```python
from build123d import *

# Parameters (mm, degrees)
F0_R     = 50
F0_R_2   = 4
F0_R_3   = 23
F2_DEPTH = 5
F4_R     = 1
F5_R     = 1


with BuildPart() as f2:
    # F0 (on Top) → F2 (new body)
    with BuildSketch(Plane.XY):
        Circle(F0_R)
        with Locations((-19.25, -33.341978)):
            Circle(F0_R_2, mode=Mode.SUBTRACT)
        with Locations((19.25, -33.341978)):
            Circle(F0_R_2, mode=Mode.SUBTRACT)
        with Locations((-38.5, 0)):
            Circle(F0_R_2, mode=Mode.SUBTRACT)
        with Locations((-19.25, 33.341978)):
            Circle(F0_R_2, mode=Mode.SUBTRACT)
        Circle(F0_R_3, mode=Mode.SUBTRACT)
        with Locations((38.5, 0)):
            Circle(F0_R_2, mode=Mode.SUBTRACT)
        with Locations((19.25, 33.341978)):
            Circle(F0_R_2, mode=Mode.SUBTRACT)
    extrude(amount=F2_DEPTH)

    # F1 (on Front) → F3 (revolve)
    with BuildSketch(Plane.XZ):
        Polygon((-26.2, 0), (-23, 0), (-23, 125), (-7, 136.203321), (-15.550504, 159.695636), (-17.154602, 159.695636), (-17.154602, 155.695636), (-19.017419, 155.263182), (-19.017419, 154.289458), (-15.842509, 151.14174), (-10.846829, 137.416221), (-26.2, 126.665815), align=None)
    revolve(axis=Axis((0, 0, 80), (0, 0, 1)))

    # F4
    f4_edges = [f2.edges().sort_by_distance(p)[0] for p in [
        (7, 0, 136.203321),
        (26.2, 0, 126.665815),
        (15.550504, 0, 159.695636),
    ]]
    fillet(f4_edges, radius=F4_R)

    # F5
    f5_edges = [f2.edges().sort_by_distance(p)[0] for p in [
        (10.846829, 0, 137.416221),
    ]]
    fillet(f5_edges, radius=F5_R)


solid = f2.part
```
CAD build for the part. Positions are in the model's coordinates, mm. A direction names the side the tool comes from. Round coordinates to 2 decimals unless told otherwise and drop trailing zeros. Loops run counter-clockwise (first coordinate to the right, second up) from the corner with the lowest first, then second, coordinate; pieces in that order, holes last. Notation, with made-up numbers: M -35.75,4.25 L 4.25,4.25 A27 ccw 4.25,20.25 Z; hole C 73,11.25 d11. An arc over 180 degrees is marked long. Use a Markdown table: item, result. Add a question column.
(1) Flat gauge pins, fed straight in: pin 1 (12 mm diameter, centred on x = -28.5, z = 32.5, fed in from +Y); pin 2 (10.5 mm diameter, centred on x = 38.5, y = 0, fed in from +Z); pin 3 (1.5 mm diameter, centred on y = 7.5, z = 100, fed in from +X). Where does each tip first touch, or does it go through?
(2) Cut at D-D (x = -32). Give the cut face in (y, z), and give its area (3 significant figures).
(3) Which spindle directions (+Z, -Z, +X, -X, +Y, -Y) get a long thin tool onto all of the face, cutting with end or side? Do faces 5 (the face through (10, -22, 0)), 6 (the face through (-11.3, -3.6, 140.2)), 7 (the face through (2.994, -22.804, 63.375)), 8 (the face through (3.411, -25.977, 64.725)). Say none if no direction does.
(4) Drill centre lines: line 1 (X direction, y = -0.5, z = 100.5); line 2 (Y direction, x = -19, z = 1); line 3 (Z direction, x = 12, y = -44.5). Where is each one in solid material? Low to high.
(5) Pull direction Y, two halves, no side cores. Call faces 1 (the face through (47.69, 15.02, 2.46)), 2 (the face through (18.383, -37.247, 2.465)), 3 (the face through (18.73, 37.31, 2.46)), 4 (the face through (22, -22, 5)): +Y half, -Y half, draft (parallel to the pull), parting line (faces both ways), or undercut.
(6) Cut at C-C (y = 0). State how many separate pieces and enclosed holes the cut face has, and give its area (3 significant figures).
(7) Cut at B-B (z = 27). Give the cut face in (x, y), and give its area (3 significant figures).
(8) Cut at A-A (x = 39). Give the cut face in (y, z).
Geometry says:
| question | item | result |
|---|---|---|
| 1 | pin 1 | stops at y = 13.42 |
| 1 | pin 2 | stops at z = 5 |
| 1 | pin 3 | stops at x = 25.32 |
| 2 | outline | M -38.42,0 L 38.42,0 L 38.42,5 L -38.42,5 Z |
| 2 | area | 384 mm² |
| 3 | face 5 | -Z, +X, -X, +Y, -Y |
| 3 | face 6 | none |
| 3 | face 7 | -Z |
| 3 | face 8 | +Z |
| 4 | line 1 | x = -26.2 to -22.99, 22.99 to 26.2 |
| 4 | line 2 | y = -46.25 to -37.33, -29.35 to -12.96, 12.96 to 29.35, 37.33 to 46.25 |
| 4 | line 3 | z = 0 to 5 |
| 5 | face 1 | parting line |
| 5 | face 2 | undercut |
| 5 | face 3 | undercut |
| 5 | face 4 | draft |
| 6 | separate pieces | 4 |
| 6 | enclosed holes | 0 |
| 6 | area | 1,240 mm² |
| 7 | outline | C 0,0 d52.4; hole C 0,0 d46 |
| 7 | area | 495 mm² |
| 8 | outline | M -31.29,0 L -3.97,0 L -3.97,5 L -31.29,5 Z; M 3.97,0 L 31.29,0 L 31.29,5 L 3.97,5 Z |
